Check sheet for the modelled part. Datum: model origin and axes. Units: mm. Round coordinates to 2 decimals unless told otherwise and drop trailing zeros. Write each loop counter-clockwise with the first axis right and the second up, starting at its lowest first coordinate (ties: lowest second). Pieces come first, ordered by that corner, then holes. Notation, with made-up numbers: (-7.5, -10.5) -> (37.5, -10.5) arc R17 cw to (37.5, 14.5) -> close; hole circle Ø7 at (61, -22.5). An arc over 180 degrees is marked (long way). One line per item, written item: value.
from build123d import *

# Parameters (mm, degrees)
F0_W     = 859
F0_H     = 2300
F1_DEPTH = 1134
F2_R     = 300
F3_R     = 100


with BuildPart() as f1:
    # F0 (on Top) → F1 (new body)
    with BuildSketch(Plane.XY):
        with Locations((345.1126752496, 1093.3118626475)):
            Rectangle(F0_W, F0_H)
    extrude(amount=F1_DEPTH)

    # F2
    f2_edges = [f1.edges().sort_by_distance(p)[0] for p in [
        (345.112675, -56.688137, 1134),
        (345.112675, 2243.311863, 1134),
    ]]
    fillet(f2_edges, radius=F2_R)

    # F3
    f3_edges = [f1.edges().sort_by_distance(p)[0] for p in [
        (774.612675, 1093.311863, 1134),
        (774.612675, 31.179828, 1046.132034),
        (774.612675, -56.688137, 417),
        (774.612675, 2155.443897, 1046.132034),
        (774.612675, 2243.311863, 417),
        (-84.387325, -56.688137, 417),
        (-84.387325, 31.179828, 1046.132034),
        (-84.387325, 1093.311863, 1134),
        (-84.387325, 2155.443897, 1046.132034),
        (-84.387325, 2243.311863, 417),
    ]]
    fillet(f3_edges, radius=F3_R)


solid = f1.part
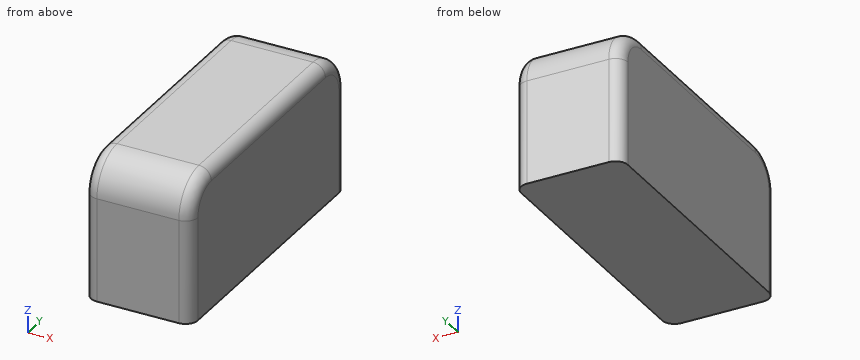
Item 1: Sectioned sample at A-A (x = 710). Enter the section's corners in (y, z).
Result set:
outline: (-50.22, 0) -> (2236.84, 0) -> (2236.84, 834) arc R293.53 ccw to (1943.31, 1127.53) -> (243.31, 1127.53) arc R293.53 ccw to (-50.22, 834) -> close
Item 2: Sectioned sample at B-B (x = -17). Enter the section's corners in (y, z).
Result set:
outline: (-51.22, 0) -> (2237.84, 0) -> (2237.84, 834) arc R294.53 ccw to (1943.31, 1128.53) -> (243.31, 1128.53) arc R294.53 ccw to (-51.22, 834) -> close
Item 3: Material ranges on line 1 along Z through (x, y) = (70.5, 107.5); line 2 along Z through (x, y) = (708, 1117.5); line 3 along Y through (x, z) = (51.5, 856), recorded low to high.
Result set:
line 1: 0 to 1101.5
line 2: 0 to 1128.26
line 3: -55.88 to 2242.5
Item 4: Depth check by flat-ended pin: pin 1 (6 mm diameter, centred on x = 614.5, y = 1953.5, fed in from +Z). Enter the tip coordinate at first touch or a pass-through.
Result set:
pin 1: z = 1133.91
